Model file for the job. Use its own axes, mm. A direction names the side the tool comes from. Coordinates: 2 decimals unless noted, no trailing zeros. Order: outer loops, then holes, each group sorted by start corner. A loop starts at its lowest first (then second) coordinate and runs counter-clockwise, first axis right, second up. Notation, with made-up numbers: (76.25, -23) -> (115.25, -23) arc R23 ccw to (115.25, -12) -> close; hole circle Ø6 at (26, -9.5). An arc over 180 degrees is marked (long way). Use CSV: the item, a comma, the result in double quotes. Start each with the question number.
(1) Pull direction X, two halves, no side cores. Call faces 1 (the flat face through (54, 20, 6)), 2 (the cylindrical face through (6.367, 2.803, 1.479)), 3 (the flat face through (50, 19, 10)), 4 (the flat face through (39, 13, 6)): pulls with the +X half, pulls with the -X half, needs draft (parallel to the pull), parting line crosses it, or undercut.
(2) Tool access for faces 5 (the flat face through (45, 13, 6)), 6 (the flat face through (50, 20, 7)), 7 (the flat face through (54.5, 17.5, 6)): list every direction of +Z, -Z, +X, -X, +Y, -Y with a clear straight run to the whole face (end or side of a thin tool).
(3) Cut at D-D on z = 1.25. Give the number of separate pieces and of enclosed holes in the cut face, plus the area to 3 significant figures.
(4) Cut at C-C on z = 6. Write the cut outline in (x, y), plus the area to 3 significant figures.
(5) Probe L1, parallel to Y at x = 5, z = 1; L2, parallel to Z at x = 57, y = 18.6; L3, parallel to Y at x = 35, z = 1.7. List the from-to ranges inside material, lowest first.
(6) Cut at A-A on x = 5. Write the cut outline in (y, z).
(7) Pin check, flat tips, straight feed: pin 1 Ø1.7 at (x, y) = (5, 2.5) entering from +Z; pin 2 Ø12 at (x, y) = (19.5, 6.5) entering from +Z; pin 3 Ø2 at (y, z) = (12.5, 6) entering from +X; pin 4 Ø5.5 at (x, y) = (50.5, 4) entering from +Z. Stop position of each tip, or through.
(8) Cut at B-B on y = 5. Write the cut outline in (x, z).
Autodesk Inventor part; units mm, degrees
ref_plane "YZ Plane" through (0, 0, 0) normal (1, 0, 0) x (0, 1, 0)
ref_plane "XZ Plane" through (0, 0, 0) normal (0, 1, 0) x (-1, 0, 0)
ref_plane "XY Plane" through (0, 0, 0) normal (0, 0, 1) x (1, 0, 0)
sketch "Sketch1" plane through (0, 0, 0) normal (0, 0, 1) x (1, 0, 0)
  line L0 (0, 0) -> (60, 0)
  line L1 (60, 0) -> (60, 15)
  line L2 (60, 15) -> (0, 15)
  line L3 (0, 15) -> (0, 0)
  dimension "d0" = 60
  dimension "d1" = 15
extrude "Extrusion1" add sketch "Sketch1" along normal blind 3
sketch "Sketch2" plane through (0, 0, 3) normal (0, 0, 1) x (1, 0, 0)
  line L0 (0, 15) -> (0, 0)
  line L1 (0, 0) -> (60, 0)
  point P0 (50, 5)
  dimension "d4" = 50
  dimension "d5" = 5
hole "Hole1" at (50, 5, 3) direction (0, 0, -1) diameter 2.8 depth 10
sketch "Sketch3" plane through (0, 0, 3) normal (0, 0, 1) x (1, 0, 0)
  point P0 (0, 0)
sketch "Sketch4" plane through (0, 0, 3) normal (0, 0, 1) x (1, 0, 0)
  circle A0 centre (50, 5) radius 2.5
  circle A1 centre (50, 5) radius 1.4
  circle A2 centre (50, 5) radius 1.4
  point P0 (0, 0)
  dimension "d13" = 5
extrude "Extrusion2" add sketch "Sketch4" along normal blind 1.5
sketch "Sketch5" plane through (0, 15, 0) normal (0, 1, 0) x (1, 0, 0)
  line L0 (0, -3) -> (60, -3)
  line L1 (60, 0) -> (45, 0)
  line L2 (45, 0) -> (45, -3)
  line L3 (45, -3) -> (60, -3)
  line L4 (60, -3) -> (60, 0)
  point P0 (0, 0)
  dimension "d16" = 15
extrude "Extrusion3" add sketch "Sketch5" along normal blind 6
sketch "Sketch6" plane through (0, 0, 3) normal (0, 0, 1) x (1, 0, 0)
  line L0 (60, 21) -> (45, 21)
  line L1 (48, 21) -> (52, 21)
  line L2 (52, 21) -> (52, 17)
  line L3 (52, 17) -> (48, 17)
  line L4 (48, 17) -> (48, 21)
  line L5 (60, 0) -> (60, 21)
  point P0 (0, 0)
  dimension "d19" = 4
  dimension "d20" = 4
  dimension "d21" = 8
extrude "Extrusion4" add sketch "Sketch6" along normal blind 7
sketch "Sketch7" plane through (0, 21, 0) normal (0, 1, 0) x (1, 0, 0)
  line L0 (48, -3) -> (48, -10)
  line L1 (52, -3) -> (52, -10)
  line L2 (48, -7) -> (52, -7)
  line L3 (52, -7) -> (52, -8.5)
  line L4 (52, -8.5) -> (48, -8.5)
  line L5 (48, -8.5) -> (48, -7)
  line L6 (52, -10) -> (48, -10)
  point P0 (0, 0)
  point P1 (50, -8.5)
  dimension "d24" = 1.5
  dimension "d25" = 1.5
extrude "Extrusion5" cut sketch "Sketch7" against normal blind 2.5 contours L2 L1 L4 L0
sketch "Sketch8" plane through (0, 0, 3) normal (0, 0, 1) x (1, 0, 0)
  line L0 (60, 21) -> (45, 21)
  line L1 (60, 21) -> (54, 21)
  line L2 (54, 21) -> (54, 17)
  line L3 (54, 17) -> (60, 17)
  line L4 (60, 17) -> (60, 21)
  point P0 (0, 0)
  dimension "d28" = 6
  dimension "d29" = 4
extrude "Extrusion6" add sketch "Sketch8" along normal blind 6
sketch "Sketch9" plane through (0, 21, 0) normal (0, 1, 0) x (1, 0, 0)
  line L0 (60, 0) -> (60, -9)
  line L1 (60, -9) -> (54, -9)
  point P0 (0, 0)
  point P1 (57, -6)
  dimension "d32" = 3
  dimension "d33" = 3
hole "Hole2" at (57, 21, 6) direction (0, -1, 0) diameter 2.8 depth 5
chamfer "Chamfer1" distance 0.75 angle 45 2 edges at (52, 17, 6.5) (48, 17, 6.5)
chamfer "Chamfer2" distance 1 angle 45 2 edges at (60, 17, 6) (54, 17, 6)
chamfer "Chamfer3" distance 3 distance2 6 1 edges at (45, 21, 1.5) measured on face at (53, 21, 1)
sketch "Sketch10" plane through (0, 0, 3) normal (0, 0, 1) x (1, 0, 0)
  line L0 (45, 15) -> (0, 15)
  line L1 (45, 15) -> (39, 15)
  line L2 (39, 15) -> (39, 11)
  line L3 (39, 11) -> (45, 11)
  line L4 (45, 11) -> (45, 15)
  point P0 (0, 0)
  dimension "d50" = 6
  dimension "d51" = 4
extrude "Extrusion7" add sketch "Sketch10" along normal blind 6
sketch "Sketch11" plane through (0, 15, 3) normal (0, 1, 0) x (1, 0, 0)
  line L0 (45, -6) -> (39, -6)
  line L1 (39, 0) -> (39, -6)
  point P0 (0, 3)
  point P1 (42, -3)
  dimension "d54" = 3
  dimension "d55" = 3
hole "Hole3" at (42, 15, 6) direction (0, -1, 0) diameter 2.8 depth 5
sketch "Sketch12" plane through (0, 0, 3) normal (0, 0, 1) x (1, 0, 0)
  line L0 (35, 12.5) -> (5, 12.5)
  line L1 (5, 12.5) -> (5, 2.5)
  line L2 (12.2868, 12.5) -> (12.2868, 15)
  line L3 (45, 15) -> (0, 15)
  line L4 (11.9839, 2.5) -> (11.9839, 0)
  line L5 (0, 0) -> (60, 0)
  line L6 (0, 15) -> (0, 0)
  dimension "d64" = 10
  dimension "d65" = 5
hole "Hole4" at (35, 12.5, 3) at (5, 12.5, 3) at (5, 2.5, 3) direction (0, 0, -1) diameter 2.8 depth 3
properties part number "probe mount 1 side"
Outcome:
1,face 1,"undercut"
1,face 2,"undercut"
1,face 3,"needs draft"
1,face 4,"pulls with the -X half"
2,face 5,"+Z, +X, +Y, -Y"
2,face 6,"-X, +Y"
2,face 7,"+Z, -Y"
3,separate pieces,"1"
3,enclosed holes,"4"
3,area,"956 mm2"
4,outline,"(39, 11) -> (40.6, 11) -> (40.6, 15) -> (39, 15) -> close; (43.4, 11) -> (45, 11) -> (45, 15) -> (43.4, 15) -> close; (48, 17.75) -> (48.75, 17) -> (51.25, 17) -> (52, 17.75) -> (52, 21) -> (48, 21) -> close; (54, 18) -> (55, 17) -> (55.6, 17) -> (55.6, 21) -> (54, 21) -> close; (58.4, 17) -> (59, 17) -> (60, 18) -> (60, 21) -> (58.4, 21) -> close"
4,area,"40.0 mm2"
5,L1,"0 to 1.1, 3.9 to 11.1, 13.9 to 15"
5,L2,"0 to 4.6, 7.4 to 9"
5,L3,"0 to 11.1, 13.9 to 15"
6,outline,"(0, 0) -> (1.1, 0) -> (1.1, 3) -> (0, 3) -> close; (3.9, 0) -> (11.1, 0) -> (11.1, 3) -> (3.9, 3) -> close; (13.9, 0) -> (15, 0) -> (15, 3) -> (13.9, 3) -> close"
7,pin 1,"through"
7,pin 2,"z = 3"
7,pin 3,"x = 45"
7,pin 4,"z = 4.5"
8,outline,"(0, 0) -> (48.6, 0) -> (48.6, 4.5) -> (47.5, 4.5) -> (47.5, 3) -> (0, 3) -> close; (51.4, 0) -> (60, 0) -> (60, 3) -> (52.5, 3) -> (52.5, 4.5) -> (51.4, 4.5) -> close"
